Autodesk Inventor part; units mm, degrees
ref_plane "YZ Plane" through (0, 0, 0) normal (1, 0, 0) x (0, 1, 0)
ref_plane "XZ Plane" through (0, 0, 0) normal (0, 1, 0) x (-1, 0, 0)
ref_plane "XY Plane" through (0, 0, 0) normal (0, 0, 1) x (1, 0, 0)
sketch "Sketch1" plane through (0, 0, 0) normal (0, 1, 0) x (-1, 0, 0)
  line L0 (18.3309, -0.0019) -> (9.1638, -15.8759)
  line L1 (9.1638, -15.8759) -> (-9.1671, -15.8741)
  line L2 (-9.1671, -15.8741) -> (-18.3309, 0.0019)
  line L3 (-18.3309, 0.0019) -> (-9.1638, 15.8759)
  line L4 (-9.1638, 15.8759) -> (9.1671, 15.8741)
  line L5 (9.1671, 15.8741) -> (18.3309, -0.0019)
  point P0 (0, 0)
  dimension "d2" = 31.75
extrude "Extrusion1" add sketch "Sketch1" along normal blind 30.1625
sketch "Sketch2" plane through (0, 30.1625, 0) normal (0, 1, 0) x (1, 0, 0)
  circle A0 centre (0, 0) radius 14.605
  dimension "d5" = 29.21
extrude "Extrusion2" add sketch "Sketch2" along normal blind 13.4938
sketch "Sketch3" plane through (0, 0, 0) normal (0, -1, 0) x (1, 0, 0)
  circle A0 centre (0, 0) radius 14.605
  dimension "d8" = 29.21
extrude "Extrusion3" add sketch "Sketch3" along normal blind 13.4938
sketch "Sketch4" plane through (0, 43.6562, 0) normal (0, 1, 0) x (1, 0, 0)
  line L0 (-7.479, 0) -> (-3.7395, 6.477)
  line L1 (-3.7395, 6.477) -> (3.7395, 6.477)
  line L2 (3.7395, 6.477) -> (7.479, 0)
  line L3 (7.479, 0) -> (3.7395, -6.477)
  line L4 (3.7395, -6.477) -> (-3.7395, -6.477)
  line L5 (-3.7395, -6.477) -> (-7.479, 0)
  point P0 (0, 0)
  point P1 (0, 0)
  dimension "d11" = 12.954
extrude "Extrusion4" cut sketch "Sketch4" against normal through all
fillet "Fillet1" radius 1.524 6 edges at (7.479, 15.0813, 0) (3.7395, 15.0813, -6.477) (-7.479, 15.0813, 0) (-3.7395, 15.0813, -6.477) (-3.7395, 15.0813, 6.477) (3.7395, 15.0813, 6.477)
sketch "Sketch5" plane through (0, 30.1625, 0) normal (0, 1, 0) x (1, 0, 0)
  circle A0 centre (0, 0) radius 14.8083
  circle A1 centre (0, 0) radius 95.25
  dimension "d15" = 190.5
extrude "Extrusion5" add sketch "Sketch5" against normal blind 30.226
sketch "Sketch6" plane through (0, 30.1625, 0) normal (0, 1, 0) x (1, 0, 0)
  circle A0 centre (0, 0) radius 95.25
  circle A1 centre (0, 0) radius 104.775
  dimension "d18" = 209.55
extrude "Extrusion6" add sketch "Sketch6" along normal blind 12.7 and the other way blind 38.1
properties part number "Wheel Hub" material "Acetal Resin, Black"
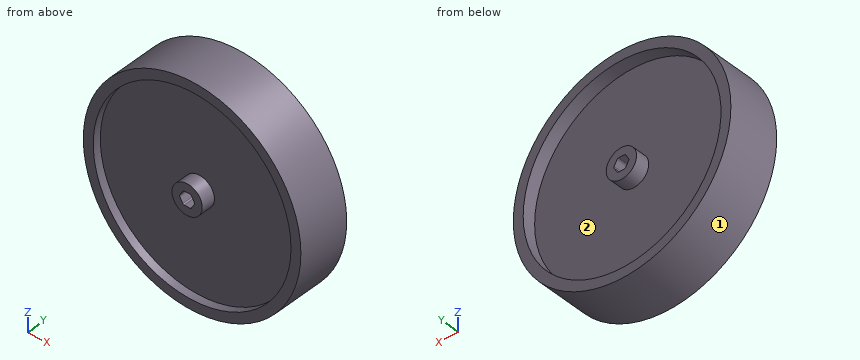
Input: part model. Units: mm. Frame: model coordinates. Face numbers are marked on the shaded views. Give positions to 0.01 mm unless a question says otherwise; leave off trailing zeros. Loops run counter-clockwise (first coordinate to the right, second up) from the corner with the lowest first, then second, coordinate; pieces in that order, holes last. Notation, with made-up numbers: M -13.75,-1 L -2.75,-1 A25 cw -2.75,22 Z; hole C 7.25,88 d2. An arc over 180 degrees is marked long. Use one line per item in the form item = value.
1. Line query: L1, parallel to X at y = 38, z = 0 (3 decimals); L2, parallel to Z at x = 0, y = 39 (3 decimals); L3, parallel to X at y = 33, z = -8. Output: solid intervals per line, ascending.
Numbers:
L1 = -104.775 to -95.25, -14.605 to -7.243, 7.243 to 14.605, 95.25 to 104.775
L2 = -104.775 to -95.25, -14.605 to -6.477, 6.477 to 14.605, 95.25 to 104.775
L3 = -104.47 to -94.91, -12.22 to 12.22, 94.91 to 104.47
2. Section query A-A, the plane y = 27.5. Return the cut outline in (x, z) (3 decimals), and give its area (3 significant figures).
Numbers:
outline = C 0,0 d209.55; hole M -7.039,-0.762 L -4.179,-5.715 A1.524 ccw -2.86,-6.477 L 2.86,-6.477 A1.524 ccw 4.179,-5.715 L 7.039,-0.762 A1.524 ccw 7.039,0.762 L 4.179,5.715 A1.524 ccw 2.86,6.477 L -2.86,6.477 A1.524 ccw -4.179,5.715 L -7.039,0.762 A1.524 ccw Z
area = 34,300 mm²
3. Section query B-B, the plane x = -82. Return the cut outline in (y, z).
Numbers:
outline = M -7.94,-65.22 L 42.86,-65.22 L 42.86,-48.46 L 30.16,-48.46 L 30.16,48.46 L 42.86,48.46 L 42.86,65.22 L -7.94,65.22 L -7.94,48.46 L -0.06,48.46 L -0.06,-48.46 L -7.94,-48.46 Z
4. First-contact query: pin 1 (5 mm diameter, centred on x = -41.5, y = 24, fed in from +Z); pin 2 (2 mm diameter, centred on x = -56.5, z = 30.5, fed in from +Y); pin 3 (1 mm diameter, centred on x = 8, y = 2.5, fed in from -Z). Flat tips, straight axial feed; report the tip coordinate or a pass-through.
Numbers:
pin_1 = 97.25
pin_2 = 30.16
pin_3 = -104.51
5. Section query C-C, the plane z = 11. Return the cut outline in (x, y), and give its area (3 significant figures).
Numbers:
outline = M -104.2,-7.94 L -94.61,-7.94 L -94.61,-0.06 L -9.91,-0.06 L -9.91,0 L -9.61,0 L -9.61,-13.49 L 9.61,-13.49 L 9.61,0 L 9.91,0 L 9.91,-0.06 L 94.61,-0.06 L 94.61,-7.94 L 104.2,-7.94 L 104.2,42.86 L 94.61,42.86 L 94.61,30.16 L 9.61,30.16 L 9.61,43.66 L -9.61,43.66 L -9.61,30.16 L -94.61,30.16 L -94.61,42.86 L -104.2,42.86 Z
area = 7,210 mm²
6. Pull-direction query (X, two-part tool) for the marked faces 1 and 2; classes: released by +X, released by -X, zero draft, split by the parting line, or undercut.
Numbers:
face_1 = split by the parting line
face_2 = undercut
7. Section query D-D, the plane z = 61.5. Return the cut outline in (x, y), and give its area (3 significant figures).
Numbers:
outline = M -84.83,-7.94 L -72.73,-7.94 L -72.73,-0.06 L 72.73,-0.06 L 72.73,-7.94 L 84.83,-7.94 L 84.83,42.86 L 72.73,42.86 L 72.73,30.16 L -72.73,30.16 L -72.73,42.86 L -84.83,42.86 Z
area = 5,630 mm²
